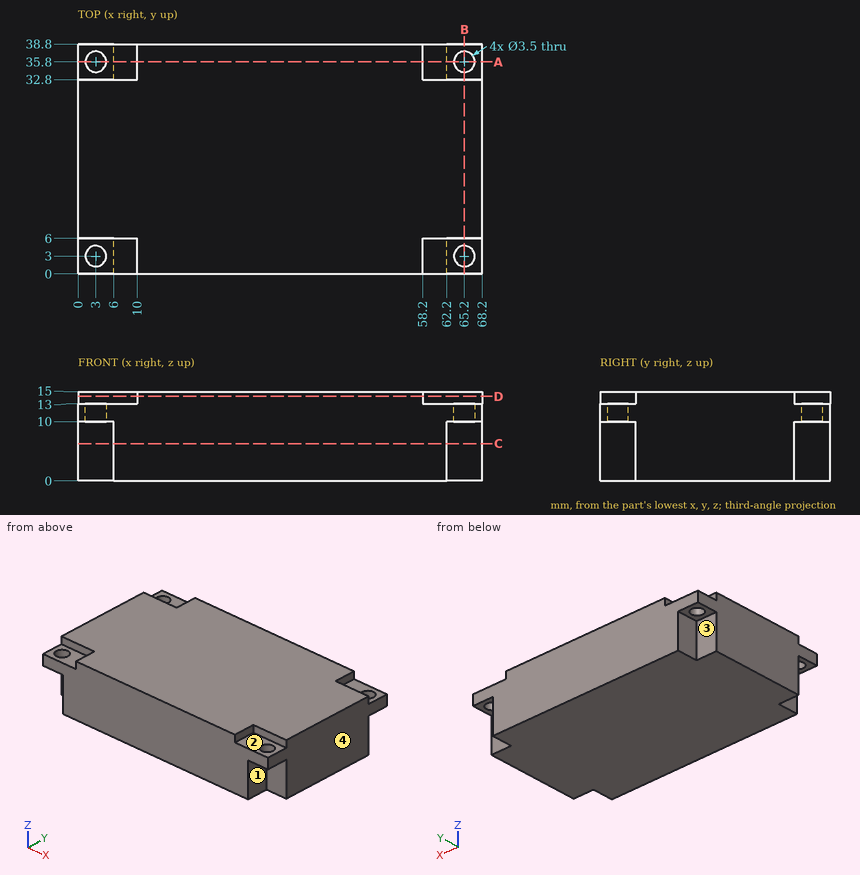
Geometry: see drawing. Coordinates: mm, zero at the bounding-box minimum. A direction names the side the tool comes from. Give positions to 0.01 mm unless a question says otherwise; leave off trailing zeros. Write each loop counter-clockwise with the first axis right and the second up, starting at its lowest first coordinate (ties: lowest second). Pieces come first, ordered by that corner, then holes. Notation, with made-up numbers: (68.25, -26) - (101.25, -26) arc R23 cw to (101.25, -9) - close; hole circle Ø8 at (50, 82.5). An arc over 180 degrees is marked (long way). Return JSON: item names as keys, results as strings. Group by question number.
1) Section C-C on z = 6.25. Return the cut outline in (x, y), plus the area to 3 significant figures.
2) First-contact query: P1, Ø6.5, axis at y = 37, z = 5.5, coming from the +X side; P2, Ø1.8, axis at x = 65, z = 5.5, coming from the -Y side; P3, Ø5.5, axis at x = 3, y = 3, coming from the -Z side; P4, Ø3, axis at x = 3, y = 35.8, coming from the +Z side. Flat tips, straight axial feed; report the tip coordinate or a pass-through.
3) Set-up query: the marked faces 1, 2, 3 and 4. Return all of +Z, -Z, +X, -X, +Y, -Y with unobstructed straight access to the full face (end or side cutting, diameter ignored); none if empty.
4) Section B-B on x = 65.2. Return the cut outline in (y, z).
5) Section D-D on z = 14.25. Return the cut outline in (x, y), plus the area to 3 significant figures.
6) Line query: line 1 (Y direction, x = 3, z = 12); line 2 (Y direction, x = 64, z = 11). Output: solid intervals per line, ascending.
7) Section A-A on y = 35.8. Return the cut outline in (x, z), plus the area to 3 significant figures.
Filled in:
{
 "1": {"outline": "(0, 6) - (6, 6) - (6, 0) - (62.2, 0) - (62.2, 6) - (68.2, 6) - (68.2, 32.8) - (62.2, 32.8) - (62.2, 38.8) - (6, 38.8) - (6, 32.8) - (0, 32.8) - close", "area": "2,500 mm^2"},
 "2": {"P1": "stops at x = 62.2", "P2": "stops at y = 6", "P3": "stops at z = 10", "P4": "passes through"},
 "3": {"face 1": "-Z, +X, -Y", "face 2": "+Z, +X, -Y", "face 3": "-Z, -X, +Y", "face 4": "+Z, -Z, +X, +Y, -Y"},
 "4": {"outline": "(0, 10) - (1.25, 10) - (1.25, 13) - (0, 13) - close; (4.75, 10) - (6, 10) - (6, 0) - (32.8, 0) - (32.8, 10) - (34.05, 10) - (34.05, 13) - (32.8, 13) - (32.8, 15) - (6, 15) - (6, 13) - (4.75, 13) - close; (37.55, 10) - (38.8, 10) - (38.8, 13) - (37.55, 13) - close"},
 "5": {"outline": "(0, 6) - (10, 6) - (10, 0) - (58.2, 0) - (58.2, 6) - (68.2, 6) - (68.2, 32.8) - (58.2, 32.8) - (58.2, 38.8) - (10, 38.8) - (10, 32.8) - (0, 32.8) - close", "area": "2,410 mm^2"},
 "6": {"line 1": "y = 0 to 1.25, 4.75 to 34.05, 37.55 to 38.8", "line 2": "y = 0 to 1.73, 4.27 to 34.53, 37.07 to 38.8"},
 "7": {"outline": "(0, 10) - (1.25, 10) - (1.25, 13) - (0, 13) - close; (4.75, 10) - (6, 10) - (6, 0) - (62.2, 0) - (62.2, 10) - (63.45, 10) - (63.45, 13) - (58.2, 13) - (58.2, 15) - (10, 15) - (10, 13) - (4.75, 13) - close; (66.95, 10) - (68.2, 10) - (68.2, 13) - (66.95, 13) - close", "area": "842 mm^2"}
}
